Can you work these out from the model? Positions are in its coordinate system, mm. A direction names the side the tool comes from. Round coordinates to 2 decimals unless told otherwise and drop trailing zeros. Write each loop counter-clockwise with the first axis right and the second up, starting at its lowest first coordinate (ties: lowest second). Pieces come first, ordered by that corner, then holes.
Q1. If we section it at D-D (y = 0.5): Please give me the cut outline in (x, z).
Q2. Please list where these lines run through material, in increasing order: line 1 along Y through (x, z) = (-1.75, -1); line 2 along Z through (x, y) = (-0.5, 2.25); line 3 along Z through (x, y) = (-1.25, 1.5).
Q3. If we section it at A-A (x = 0.25): Please give me the cut outline in (y, z), plus the area to 3 significant figures.
Q4. I'm going to push flat-ended pins straight in: pin 1 Ø1 at (x, y) = (-0.5, 3) entering from +Z; pin 2 Ø1.5 at (x, z) = (1, -2) entering from -Y; pin 3 Ø1.6 at (x, y) = (-0.5, 5) entering from -Z. Where does each tip first touch, or does it pass through?
Q5. If we section it at C-C (y = 5): Please give me the cut outline in (x, z).
Q6. If we section it at B-B (z = 1.5): Please give me the cut outline in (x, y).
Q7. For faces 1 (the flat face through (1.51, 4.35, -0.85)), 2 (the flat face through (1.5, 8, -1.4)), 3 (the flat face through (0, 4, 1.732)), which set-ups out of +Z, -Z, +X, -X, +Y, -Y let a thin tool reach every point of the face, with its end or its side?
from build123d import *

# Parameters (mm, degrees)
BOSS_EXTRUDE1_DEPTH = 8
CHAMFER2_SIZE       = 0.8
BOSS_EXTRUDE2_DEPTH = 1


with BuildPart() as part:
    # Sketch1 → Boss-Extrude1 (new body)
    with BuildSketch(Plane(origin=(0, 0, 0), x_dir=(1, 0, 0), z_dir=(0, 1, 0))):
        Polygon((2, 0), (1, 1.732050808), (-1, 1.732050808), (-2, 0), (-1, -1.732050808), (1, -1.732050808), align=None)
    extrude(amount=BOSS_EXTRUDE1_DEPTH)

    # Chamfer2
    chamfer2_edges = [part.edges().sort_by_distance(p)[0] for p in [
        (0, 0, 1.732050808),
        (-1.5, 0, 0.866025404),
        (-1.5, 0, -0.866025404),
        (0, 0, -1.732050808),
        (1.5, 0, -0.866025404),
        (1.5, 0, 0.866025404),
    ]]
    chamfer(chamfer2_edges, length=CHAMFER2_SIZE)

    # Sketch2 → Boss-Extrude2 (add)
    with BuildSketch(Plane(origin=(0, 8, 0), x_dir=(1, 0, 0), z_dir=(0, 1, 0))):
        Polygon((-3.464101615, 0), (-1.732050808, -3), (1.732050808, -3), (3.464101615, 0), (1.732050808, 3), (-1.732050808, 3), align=None)
    extrude(amount=BOSS_EXTRUDE2_DEPTH)


solid = part.part
A:
1. outline: (-1.65, 0) - (-0.83, -1.43) - (0.83, -1.43) - (1.65, 0) - (0.83, 1.43) - (-0.83, 1.43) - close
2. line 1: y = 8 to 9
2. line 2: z = -1.73 to 1.73
2. line 3: z = -1.3 to 1.3
3. outline: (0, -0.93) - (0.8, -1.73) - (8, -1.73) - (8, -3) - (9, -3) - (9, 3) - (8, 3) - (8, 1.73) - (0.8, 1.73) - (0, 0.93) - close
3. area: 33.1 mm2
4. pin 1: stops at z = 1.73
4. pin 2: stops at y = 0.36
4. pin 3: stops at z = -1.73
5. outline: (-2, 0) - (-1, -1.73) - (1, -1.73) - (2, 0) - (1, 1.73) - (-1, 1.73) - close
6. outline: (-2.6, 8) - (-1.13, 8) - (-1.13, 0.8) - (-0.87, 0.57) - (0.87, 0.57) - (1.13, 0.8) - (1.13, 8) - (2.6, 8) - (2.6, 9) - (-2.6, 9) - close
7. face 1: -Z, +X, -Y
7. face 2: -Y
7. face 3: +Z, +X, -X, -Y
